Geometry: final body of the model. Coordinates: model frame, mm. A direction names the side the tool comes from. Give positions to 0.01 mm unless a question says otherwise; leave off trailing zeros. Loops run counter-clockwise (first coordinate to the right, second up) from the corner with the lowest first, then second, coordinate; pieces in that order, holes last.
1. Section A-A, the plane z = 5.25. Output: boundary loops of the cut face in (x, y), then the cut area to 3 significant figures.
2. First-contact query: P1, Ø1.5, axis at y = 15, z = -1.5, coming from the -X side; P2, Ø5, axis at x = 3, y = 10, coming from the +Z side; P3, Ø2, axis at x = -2, y = 6, coming from the -Z side. Flat tips, straight axial feed; report the tip coordinate or a pass-through.
3. Section B-B, the plane y = 21.5. Output: boundary loops of the cut face in (x, z).
4. Draft query along Y for faces 3 (the face through (-1.2, 0, 2.5)), 4 (the face through (2, 4.357, -5)), 5 (the face through (2, 8.421, -5)), 6 (the face through (5.666, 19.583, -0.744)). Return one class per face: +Y half, -Y half, draft (parallel to the pull), parting line (faces both ways), or undercut.
5. Material intervals for line 1 along Y through (x, z) = (-4, -3.5); line 2 along X through (y, z) = (17.75, 0); line 3 along X through (y, z) = (8, 0) (3 decimals), sorted ascending.
6. Access query for faces 1 (the face through (2, 10.453, -5)), 2 (the face through (5.666, 7.391, -0.744)). Directions: +Z, -Z, +X, -X, +Y, -Y. A direction counts if a zero-diameter tool reaches every point of the face in a straight line with its end or side. Return the directions, or none.
from build123d import *

# Parameters (mm, degrees)
SKETCH1_R           = 5.715
SKETCH1_R_2         = 2.54
BOSS_EXTRUDE1_DEPTH = 25.4
SKETCH3_W           = 0.779816736
SKETCH3_H           = 2.032


with BuildPart() as part:
    # Sketch1 → Boss-Extrude1 (new body)
    with BuildSketch(Plane(origin=(0, 0, 0), x_dir=(1, 0, 0), z_dir=(0, 1, 0))):
        with Locations(Location((0, 0, 0), (0, 0, 270))):
            Circle(SKETCH1_R)
        with Locations(Location((0, 0, 0), (0, 0, 270))):
            Circle(SKETCH1_R_2, mode=Mode.SUBTRACT)
    extrude(amount=BOSS_EXTRUDE1_DEPTH)

    # Sketch3 → Cut-Revolve2 (revolve, cut)
    with BuildSketch(Plane(origin=(0, 0, 0), x_dir=(0, 0, -1), z_dir=(1, 0, 0))):
        with Locations((5.325091632, 5.373385887)):
            Rectangle(SKETCH3_W, SKETCH3_H)
        with Locations((5.325091632, 9.437385887)):
            Rectangle(SKETCH3_W, SKETCH3_H)
        with Locations((5.325091632, 13.501385887)):
            Rectangle(SKETCH3_W, SKETCH3_H)
        with Locations((5.325091632, 17.565385887)):
            Rectangle(SKETCH3_W, SKETCH3_H)
        with Locations((5.325091632, 21.629385887)):
            Rectangle(SKETCH3_W, SKETCH3_H)
    revolve(axis=Axis((0, 0, 0), (0, 1, 0)), mode=Mode.SUBTRACT)


solid = part.part
Answers below:
1. outline: (-2.26, 0) - (2.26, 0) - (2.26, 4.36) - (-2.26, 4.36) - close; (-2.26, 6.39) - (2.26, 6.39) - (2.26, 8.42) - (-2.26, 8.42) - close; (-2.26, 10.45) - (2.26, 10.45) - (2.26, 12.49) - (-2.26, 12.49) - close; (-2.26, 14.52) - (2.26, 14.52) - (2.26, 16.55) - (-2.26, 16.55) - close; (-2.26, 18.58) - (2.26, 18.58) - (2.26, 20.61) - (-2.26, 20.61) - close; (-2.26, 22.65) - (2.26, 22.65) - (2.26, 25.4) - (-2.26, 25.4) - close
1. area: 68.8 mm2
2. P1: stops at x = -5.67
2. P2: stops at z = 5.69
2. P3: stops at z = -5.61
3. outline: circle Ø9.87 at (0, 0); hole circle Ø5.08 at (0, 0)
4. face 3: -Y half
4. face 4: undercut
4. face 5: undercut
4. face 6: draft
5. line 1: y = 0 to 4.36, 6.39 to 8.42, 10.45 to 12.49, 14.52 to 16.55, 18.58 to 20.61, 22.65 to 25.4
5. line 2: x = -4.94 to -2.54, 2.54 to 4.94
5. line 3: x = -5.715 to -2.54, 2.54 to 5.715
6. face 1: none
6. face 2: +Y, -Y
